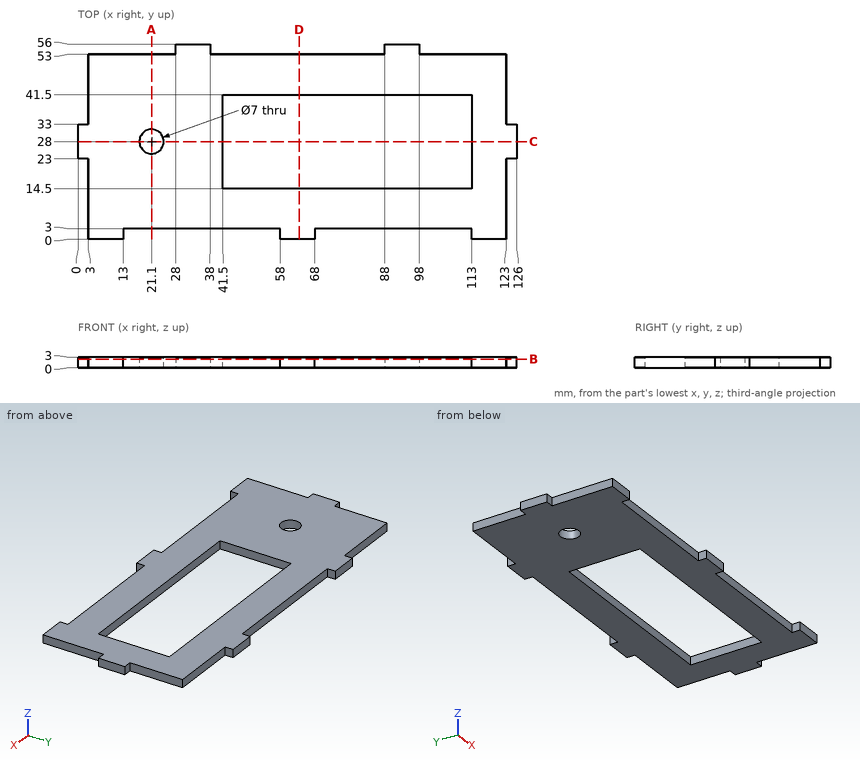
Job drawing, mm, ordinate dimensions from the low corner. One solid piece. Coordinates: 2 decimals unless noted, no trailing zeros. Order: outer loops, then holes, each group sorted by start corner. A loop starts at its lowest first (then second) coordinate and runs counter-clockwise, first axis right, second up. Notation, with made-up numbers: M 0,-31 L 5,-31 A15 ccw 5,-3 Z; hole C -8.5,-37.5 d7. An arc over 180 degrees is marked long. Answer as CSV lines item,"result".
(1) Flat gauge pins, fed straight in: pin 1 (6 mm diameter, centred on x = 102.5, y = 16.5, fed in from -Z); pin 2 (1.5 mm diameter, centred on y = 54.5, z = 2, fed in from +X); pin 3 (3 mm diameter, centred on x = 110, y = 17, fed in from -Z); pin 4 (1.5 mm diameter, centred on x = 71.5, z = 1, fed in from +Y). Where does each tip first touch, or does it go through?
Geometry says:
pin 1,"stops at z = 0"
pin 2,"stops at x = 98"
pin 3,"passes through"
pin 4,"stops at y = 53"
(2) Wall check: line 1 along Y through (x, z) = (106, 1.3); line 2 along X through (y, z) = (32.5, 0.35); line 3 along Y through (x, z) = (21.1, 1). Give the ranges that are in metal, low to high.
Geometry says:
line 1,"y = 3 to 14.5, 41.5 to 53"
line 2,"x = 0 to 41.5, 113 to 126"
line 3,"y = 3 to 24.5, 31.5 to 53"
(3) Band-saw the part on D-D, the plane x = 63.5. List the corners of the cut face in (y, z).
Geometry says:
outline,"M 0,0 L 14.5,0 L 14.5,3 L 0,3 Z; M 41.5,0 L 53,0 L 53,3 L 41.5,3 Z"
(4) Band-saw the part on C-C, the plane y = 28. List the corners of the cut face in (x, z), then the cut area to 4 significant figures.
Geometry says:
outline,"M 0,0 L 17.6,0 L 17.6,3 L 0,3 Z; M 24.6,0 L 41.5,0 L 41.5,3 L 24.6,3 Z; M 113,0 L 126,0 L 126,3 L 113,3 Z"
area,"142.5 mm2"
(5) Band-saw the part on A-A, the plane x = 21.1. List the corners of the cut face in (y, z).
Geometry says:
outline,"M 3,0 L 24.5,0 L 24.5,3 L 3,3 Z; M 31.5,0 L 53,0 L 53,3 L 31.5,3 Z"
(6) Band-saw the part on B-B, the plane z = 2.4. State how many separate pieces and enclosed holes the cut face has, then the cut area to 3 significant figures.
Geometry says:
separate pieces,"1"
enclosed holes,"2"
area,"4,240 mm2"
